Job drawing, mm, ordinate dimensions from the low corner. One solid piece. Give positions to 0.01 mm unless a question says otherwise; leave off trailing zeros. Order: outer loops, then holes, each group sorted by start corner. A loop starts at its lowest first (then second) coordinate and runs counter-clockwise, first axis right, second up. Notation, with made-up numbers: (83, 75) -> (129, 75) arc R28 cw to (129, 107) -> close; hole circle Ø3 at (-9.5, 77.5). An arc over 180 degrees is marked (long way). Use CSV: the item, a comma, the result in double quotes. Start each with the question number.
1. Wall check: line 1 (X direction, y = 27, z = 25); line 2 (X direction, y = 36.5, z = 13); line 3 (Z direction, x = 91, y = 24.5) (3 decimals). Give the ranges that are in metal, low to high. Write a range as from..to.
2. Cut at D-D on y = 6. List the corners of the cut face in (x, z), then the cut area to 3 significant figures.
3. Cut at B-B on x = 251. List the corners of the cut face in (y, z).
4. Cut at A-A on y = 25. List the corners of the cut face in (x, z).
5. Cut at C-C on z = 45. List the corners of the cut face in (x, y), then the cut area to 3 significant figures.
6. Drop flat-ended pins along their axis: pin 1 (3 mm diameter, centred on x = 69, y = 15, fed in from -Z); pin 2 (5.5 mm diameter, centred on x = 10, z = 25, fed in from +Y); pin 3 (4 mm diameter, centred on x = 341, z = 45, fed in from +Y); pin 4 (3.5 mm diameter, centred on x = 440, z = 25, fed in from -Y). Give the stop position or say it passes through.
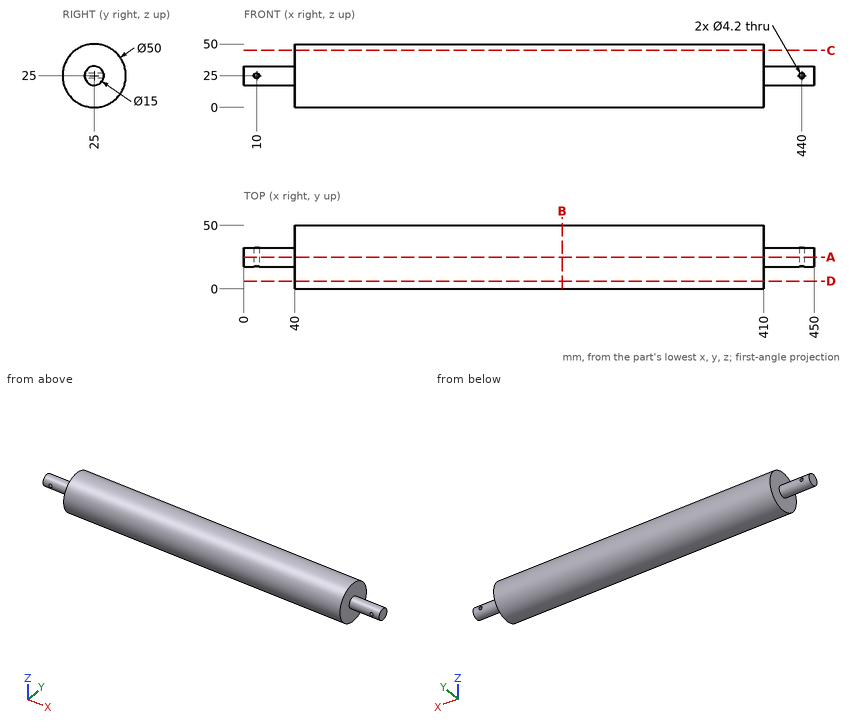
Verdict:
1,line 1,"0..7.9, 12.1..437.9, 442.1..450"
1,line 2,"40..410"
1,line 3,"0.005..49.995"
2,outline,"(40, 8.75) -> (410, 8.75) -> (410, 41.25) -> (40, 41.25) -> close"
2,area,"12,000 mm^2"
3,outline,"circle Ø50 at (25, 25)"
4,outline,"(0, 17.5) -> (40, 17.5) -> (40, 0) -> (410, 0) -> (410, 17.5) -> (450, 17.5) -> (450, 32.5) -> (410, 32.5) -> (410, 50) -> (40, 50) -> (40, 32.5) -> (0, 32.5) -> close; hole circle Ø4.2 at (10, 25); hole circle Ø4.2 at (440, 25)"
5,outline,"(40, 10) -> (410, 10) -> (410, 40) -> (40, 40) -> close"
5,area,"11,100 mm^2"
6,pin 1,"z = 1.49"
6,pin 2,"y = 32.5"
6,pin 3,"y = 42.35"
6,pin 4,"through"
